Here's how the part is built. I have some questions about the finished solid (model axes, mm). Give positions to 0.01 mm unless a question says otherwise; leave off trailing zeros. Order: outer loops, then holes, each group sorted by start corner. A loop starts at its lowest first (then second) coordinate and runs counter-clockwise, first axis right, second up. Notation, with made-up numbers: M 36,29.5 L 86,29.5 A20 cw 86,42.5 Z; hole C 56,10 d5. An arc over 180 degrees is marked long. One line per item, written item: value. Start each with the question number.
Autodesk Inventor part; units mm, degrees
ref_plane "YZ Plane" through (0, 0, 0) normal (1, 0, 0) x (0, 1, 0)
ref_plane "XZ Plane" through (0, 0, 0) normal (0, 1, 0) x (-1, 0, 0)
ref_plane "XY Plane" through (0, 0, 0) normal (0, 0, 1) x (1, 0, 0)
sketch "Sketch1" plane through (0, 0, 0) normal (0, 0, 1) x (1, 0, 0)
  line L0 (0, 0) -> (200, 0)
  line L1 (200, 0) -> (200, 150)
  line L2 (200, 150) -> (0, 150)
  line L3 (0, 150) -> (0, 0)
  dimension "d0" = 200
  dimension "d1" = 150
extrude "Extrusion1" add sketch "Sketch1" along normal blind 3
sketch "Sketch2" plane through (0, 0, 3) normal (0, 0, 1) x (1, 0, 0)
  line L0 (0, 0) -> (40, 0)
  line L1 (0, 0) -> (200, 0)
  line L2 (40, 0) -> (40, 3)
  line L3 (40, 3) -> (80, 3)
  line L4 (80, 3) -> (80, 0)
  line L5 (80, 0) -> (120, 0)
  line L6 (0, 150) -> (0, 0)
  line L7 (0, 75) -> (200, 75)
  line L8 (200, 0) -> (200, 150)
  line L9 (120, 0) -> (120, 3)
  line L10 (120, 3) -> (160, 3)
  line L11 (160, 3) -> (160, 0)
  line L12 (40, 0) -> (80, 0)
  line L13 (120, 0) -> (160, 0)
  line L14 (200, 150) -> (0, 150)
  line L15 (0, 150) -> (0, 120)
  line L16 (0, 120) -> (3, 120)
  line L17 (3, 120) -> (3, 90)
  line L18 (3, 90) -> (0, 90)
  line L19 (0, 90) -> (0, 60)
  line L20 (0, 60) -> (3, 60)
  line L21 (3, 60) -> (3, 30)
  line L22 (3, 30) -> (0, 30)
  line L23 (0, 30) -> (0, 0)
  line L24 (100, 150) -> (100, 0)
  line L25 (0, 60) -> (0, 30)
  line L26 (0, 120) -> (0, 90)
  line L27 (200, 120) -> (197, 120)
  line L28 (197, 120) -> (197, 90)
  line L29 (197, 90) -> (200, 90)
  line L30 (200, 90) -> (200, 60)
  line L31 (200, 60) -> (197, 60)
  line L32 (197, 60) -> (197, 30)
  line L33 (197, 30) -> (200, 30)
  line L34 (200, 60) -> (200, 30)
  line L35 (200, 120) -> (200, 90)
  line L36 (40, 150) -> (40, 147)
  line L37 (40, 147) -> (80, 147)
  line L38 (80, 147) -> (80, 150)
  line L39 (80, 150) -> (120, 150)
  line L40 (120, 150) -> (120, 147)
  line L41 (120, 147) -> (160, 147)
  line L42 (160, 147) -> (160, 150)
  line L43 (40, 150) -> (80, 150)
  line L44 (120, 150) -> (160, 150)
  dimension "d4" = 40
  dimension "d6" = 3
  dimension "d7" = 40
  dimension "d8" = 40
  dimension "d19" = 40
  dimension "d20" = 30
  dimension "d21" = 3
  dimension "d22" = 30
  dimension "d23" = 30
  dimension "d24" = 30
extrude "Extrusion2" cut sketch "Sketch2" against normal blind 3 contours L2 L3 L4 L1 | L6 L20 L21 L22 | L9 L10 L11 L1 | L6 L16 L17 L18 | L8 L33 L32 L31 | L29 L28 L27 L8 | L14 L42 L41 L40 | L38 L37 L36 L14
properties part number "TAPA"
Item 1: I want a section at B-B on y = 109.5. Write out the boundary of the cut face in (x, z), plus the area to 3 significant figures.
Item 2: Will these pins go through, and if not, where does the flat tip stop? P1, Ø1.5, axis at y = 112, z = 2, coming from the -X side; P2, Ø1.5, axis at x = 55.5, z = 1, coming from the -Y side; P3, Ø0.9, axis at y = 38, z = 1, coming from the +X side.
Item 3: I want a section at A-A on x = 141. Write out the boundary of the cut face in (y, z).
Item 4: Please list where these lines run through material, in increasing order: probe 1 along X at (y, z) = (119, 0.6); probe 2 along Y at (x, z) = (79, 0.8). Write a range as [from, to].
Answer below:
1. outline: M 3,0 L 197,0 L 197,3 L 3,3 Z
1. area: 582 mm²
2. P1: stops at x = 3
2. P2: stops at y = 3
2. P3: stops at x = 197
3. outline: M 3,0 L 147,0 L 147,3 L 3,3 Z
4. probe 1: x = [3, 197]
4. probe 2: y = [3, 147]
